Source: three-view drawing plus pictorial views. Frame: mm from the lowest corner of the part. A direction names the side the tool comes from. Give positions to 0.01 mm unless a question says otherwise; leave off trailing zeros. Order: outer loops, then holes, each group sorted by start corner. A loop starts at its lowest first (then second) coordinate and runs counter-clockwise, first axis right, second up. Notation, with made-up numbers: (-24, -40) -> (-12, -40) arc R12 ccw to (-12, -19) -> close; hole circle Ø11 at (-12, 6). An arc over 180 degrees is marked (long way). Write item = value, one per line.
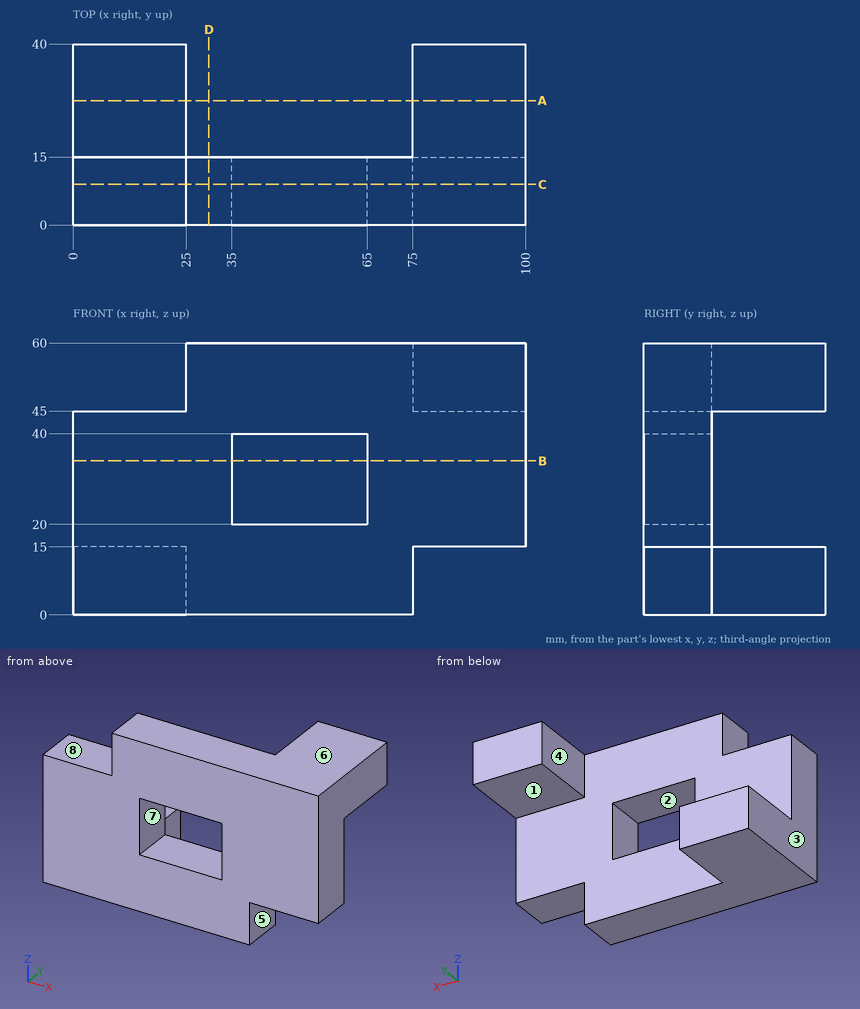
1) Section query B-B (z = 34). Output: boundary loops of the cut face in (x, y), plus the area to 3 significant figures.
Check sheet entries:
outline = (0, 0) -> (35, 0) -> (35, 15) -> (0, 15) -> close; (65, 0) -> (100, 0) -> (100, 15) -> (65, 15) -> close
area = 1,050 mm²
2) First-contact query: P1, Ø7.5, axis at x = 93, y = 10.5, coming from the -Z side; P2, Ø2, axis at x = 25.5, y = 17, coming from the -Z side; P3, Ø10, axis at x = 85.5, z = 20, coming from the +Y side; P4, Ø12, axis at x = 14, y = 8, coming from the +Z side. Flat tips, straight axial feed; report the tip coordinate or a pass-through.
Check sheet entries:
P1 = 15
P2 = 0
P3 = 15
P4 = 45
3) Reachability of the marked faces 4, 5, 6, 7 and 8 from +Z, -Z, +X, -X, +Y, -Y: full face, straight path, thin tool, end or side. Return the list, or none.
Check sheet entries:
face_4 = +Z, -Z, -X, +Y
face_5 = -Z, +X, +Y, -Y
face_6 = +Z, +X, -X, +Y, -Y
face_7 = +Y, -Y
face_8 = +Z, -X, +Y, -Y
4) Section query D-D (x = 30). Output: boundary loops of the cut face in (y, z), plus the area to 3 significant figures.
Check sheet entries:
outline = (0, 0) -> (15, 0) -> (15, 60) -> (0, 60) -> close
area = 900 mm²
5) Section query A-A (y = 27.5). Output: boundary loops of the cut face in (x, z).
Check sheet entries:
outline = (0, 0) -> (25, 0) -> (25, 15) -> (0, 15) -> close; (75, 45) -> (100, 45) -> (100, 60) -> (75, 60) -> close
6) Mould query, pull axis X, two halves, no side actions, for the marked faces 1, 2 and 3. Classes: +X half, -X half, draft (parallel to the pull), parting line (faces both ways), or undercut.
Check sheet entries:
face_1 = draft
face_2 = undercut
face_3 = -X half
7) Line query: line 1 (Z direction, x = 60, y = 13); line 2 (X direction, y = 13, z = 26); line 3 (Y direction, x = 8, z = 44.5). Output: solid intervals per line, ascending. Write a range as from..to.
Check sheet entries:
line_1 = 0..20, 40..60
line_2 = 0..35, 65..100
line_3 = 0..15
8) Section query C-C (y = 9). Output: boundary loops of the cut face in (x, z), plus the area to 3 significant figures.
Check sheet entries:
outline = (0, 0) -> (75, 0) -> (75, 15) -> (100, 15) -> (100, 60) -> (25, 60) -> (25, 45) -> (0, 45) -> close; hole (35, 20) -> (65, 20) -> (65, 40) -> (35, 40) -> close
area = 4,650 mm²
